Autodesk Inventor part; units mm, degrees
ref_plane "YZ Plane" through (0, 0, 0) normal (1, 0, 0) x (0, 1, 0)
ref_plane "XZ Plane" through (0, 0, 0) normal (0, 1, 0) x (-1, 0, 0)
ref_plane "XY Plane" through (0, 0, 0) normal (0, 0, 1) x (1, 0, 0)
sketch "Эскиз1" plane through (0, 0, 0) normal (0, 0, 1) x (1, 0, 0)
  circle A0 centre (4.9, 18.1) radius 0.455
  circle A1 centre (4.9, 18.1) radius 0.7
  line L0 (6.3, 16.875) -> (6.3, 18.1)
  line L1 (0, 22.5) -> (7, 22.5)
  line L2 (7, 22.5) -> (7, 21.25)
  line L3 (7, 21.25) -> (1.75, 21.25)
  line L4 (0, 0) -> (9.5856, 0)
  line L5 (0, 22.5) -> (0, 18.1)
  line L6 (0, 18.1) -> (1.75, 17.75)
  line L7 (1.75, 17.75) -> (4.9, 16)
  line L8 (4.9, 16) -> (6.3, 16.875)
  line L9 (4.9, 16) -> (0, 16) construction
  line L10 (0, 18) -> (0, -3)
  line L11 (-1.9171, 0) -> (11.5027, 0)
  line L12 (4.2, 18.1) -> (1.75, 18.59)
  line L13 (1.75, 18.59) -> (1.75, 21.25)
  line L14 (6.3, 18.1) -> (5.6, 18.1)
  dimension "d0" = 45
  dimension "d1" = 33.75
  dimension "d2" = 1.25
  dimension "d3" = 0.91
  dimension "d4" = 1.4
  dimension "d5" = 32
  dimension "d6" = 35.5
  dimension "d7" = 36.2
  dimension "d8" = 4.9
  dimension "d9" = 6.3
  dimension "d10" = 7
  dimension "d12" = 1.75
revolve "Базовый элемент" add sketch "Эскиз1" angle 360 about axis through (0, 0, 0) along (1, 0, 0) contours L14 L0 L8 L7 L6 L5 L1 L2 L3 L13 L12 A1
revolve "Пружинные1" add sketch "Эскиз1" angle 360 about axis through (0, 0, 0) along (1, 0, 0) contours A0 | A1
fillet "Сопряжение1" radius 0.4 3 edges at (7, -22.5, 0) (1.75, -21.25, 0) (0, -22.5, 0)
equation "\"d0\" = SD2"
equation "\"d1\" = ABDM"
equation "\"d3\" = SPDI"
equation "\"d4\" = SPDA"
equation "\"d5\" = NND"
equation "\"d6\" = TKDM"
equation "\"d7\" = HLDM"
equation "\"d8\" = SPDST"
equation "\"d9\" = SDI"
equation "\"d10\" = SWDT"
equation "\"d12\" = SD"
equation "\"d11\" = RR"
equation "\"SD2\" = 45"
equation "\"SWDT\" = 7"
equation "\"RR\" = 0.4"
equation "\"SD\" = 1.75"
equation "\"NND\" = 32"
equation "\"SPDA\" = 1.4"
equation "\"SPDI\" = 0.91"
equation "\"TKDM\" = 35.5"
equation "\"HLDM\" = 36.2"
equation "\"ABDM\" = 33.75"
equation "\"SDI\" = 6.3"
equation "\"SPDST\" = 4.9"
equation "\"LAB\" = 0.35"
properties part number "Манжет 1-32x45x7 ГОСТ 8752-79" material "Резина"
CAD build for the part. Positions are in the model's coordinates, mm. A direction names the side the tool comes from. Round coordinates to 2 decimals unless told otherwise and drop trailing zeros. Write each loop counter-clockwise with the first axis right and the second up, starting at its lowest first coordinate (ties: lowest second). Pieces come first, ordered by that corner, then holes. Notation, with made-up numbers: M 50.5,-0.5 L 77.5,-0.5 A35 cw 77.5,31.5 Z; hole C -15,18.5 d3. An arc over 180 degrees is marked long. Put each result on its own line as item: value. Start each with the question number.
1) Drill centre lines: probe 1 along Y at (x, z) = (5.75, 2.5); probe 2 along Y at (x, z) = (4.5, -3); probe 3 along Z at (x, y) = (4.9, 0). Where is each one in solid material? Low to high. Write a range as [from, to].
2) Saw through at C-C, the plane x = 3. Write the cut outline in (y, z), and give its area (3 significant figures).
3) 3-axis set-ups, long thin cutter, end or side, ignore diameter. For faces 1 (the cylindrical face through (4.541, -16.863, 12.93)), 2 (the flat face through (1.75, -19, -1)), 3 (the flat face through (7, -12, 18)): which of +Z, -Z, +X, -X, +Y, -Y reach the whole face in a straight line?
4) Pull direction X, two halves, no side cores. Call faces 4 (the conical face through (4.703, 15.366, -4.839)), 5 (the conical face through (4.047, 8.366, 16.085)), 6 (the flat face through (6.3, 5.3, 16.2)): pulls with the +X half, pulls with the -X half, needs draft (parallel to the pull), parting line crosses it, or undercut.
5) Pin check, flat tips, straight feed: pin 1 Ø2 at (x, y) = (4, -1.5) entering from -Z; pin 2 Ø21 at (y, z) = (5, -6) entering from +X; pin 3 Ø1 at (x, z) = (5.5, -15) entering from -Y. Stop position of each tip, or through.
Resolved:
1. probe 1: [-22.36, -21.1], [-17.93, -16.34], [16.34, 17.93], [21.1, 22.36]
1. probe 2: [-22.3, -21.04], [-18.43, -15.94], [15.94, 18.43], [21.04, 22.3]
1. probe 3: [-22.5, -21.25], [-18.8, -16], [16, 18.8], [21.25, 22.5]
2. outline: C 0,0 d45; C 0,0 d36.68; hole C 0,0 d42.5; hole C 0,0 d34.11
2. area: 315 mm²
3. face 1: +X
3. face 2: none
3. face 3: +Z, -Z, +X, +Y, -Y
4. face 4: pulls with the -X half
4. face 5: undercut
4. face 6: pulls with the +X half
5. pin 1: z = -22.49
5. pin 2: x = 6.3
5. pin 3: y = -17.2
